```python
from build123d import *

# Parameters (mm, degrees)
BOSS_EXTRUDE1_DEPTH      = 60.1
BOSS_EXTRUDE1_DEPTH_BACK = 60.1
CUT_EXTRUDE3_DEPTH       = 86.526286164
CUT_EXTRUDE3_DEPTH_BACK  = 86.526286164
SKETCH2_R                = 3.34
CUT_EXTRUDE5_DEPTH       = 86.526286164
SKETCH8_R                = 5.08
CUT_EXTRUDE6_DEPTH       = 6.858


with BuildPart() as part:
    # Sketch5 → Boss-Extrude1 (new, two sides: drawn at the far end of the back side and taken through both)
    with BuildSketch(Plane(origin=(0, 0, 0), x_dir=(0, 0, -1), z_dir=(1, 0, 0)).offset(-BOSS_EXTRUDE1_DEPTH_BACK)):
        Polygon((60.1, 0), (-60.1, 0), (-54.75, 9.525), (54.75, 9.525), align=None)
    extrude(amount=BOSS_EXTRUDE1_DEPTH + BOSS_EXTRUDE1_DEPTH_BACK)

    # Sketch6 → Cut-Extrude3 (cut, two sides: drawn at the far end of the back side and taken through both)
    with BuildSketch(Plane.XY.offset(-CUT_EXTRUDE3_DEPTH_BACK)):
        Polygon((-54.75, 9.525), (-60.1, 0), (-60.1, 9.525), align=None)
        Polygon((60.1, 9.525), (54.75, 9.525), (60.1, 0), align=None)
    extrude(amount=CUT_EXTRUDE3_DEPTH + CUT_EXTRUDE3_DEPTH_BACK, mode=Mode.SUBTRACT)

    # Sketch2 → Cut-Extrude5 (cut, through all)
    with BuildSketch(Plane(origin=(0, 0, 0), x_dir=(1, 0, 0), z_dir=(0, 1, 0))):
        with Locations(Location((-25, 25, 0), (0, 0, 270))):
            Circle(SKETCH2_R)
        with Locations(Location((25, 25, 0), (0, 0, 270))):
            Circle(SKETCH2_R)
        with Locations(Location((25, -25, 0), (0, 0, 270))):
            Circle(SKETCH2_R)
        with Locations(Location((-25, -25, 0), (0, 0, 270))):
            Circle(SKETCH2_R)
        Polygon((-39.357563441, 0), (0, 39.357563441), (39.357563441, 0), (0, -39.357563441), align=None)
    extrude(amount=CUT_EXTRUDE5_DEPTH, mode=Mode.SUBTRACT)

    # Sketch8 → Cut-Extrude6 (cut)
    with BuildSketch(Plane.XZ):
        with Locations(Location((-25, 25, 0), (0, 0, 270))):
            Circle(SKETCH8_R)
        with Locations(Location((25, 25, 0), (0, 0, 270))):
            Circle(SKETCH8_R)
        with Locations(Location((25, -25, 0), (0, 0, 270))):
            Circle(SKETCH8_R)
        with Locations(Location((-25, -25, 0), (0, 0, 270))):
            Circle(SKETCH8_R)
    extrude(amount=-CUT_EXTRUDE6_DEPTH, mode=Mode.SUBTRACT)


solid = part.part
```
Here's how the part is built. I have some questions about the finished solid (model axes, mm). A direction names the side the tool comes from. Round coordinates to 2 decimals unless told otherwise and drop trailing zeros. Loops run counter-clockwise (first coordinate to the right, second up) from the corner with the lowest first, then second, coordinate; pieces in that order, holes last. Notation, with made-up numbers: (71, 74) -> (93, 74) arc R37 cw to (93, 112) -> close; hole circle Ø9 at (-17.5, 44). An arc over 180 degrees is marked (long way). Answer as CSV lines item,"result". Start each with the question number.
1. If we mould it in two halves opening along X, with no side actions, what happens to faces 4 (the face through (-37, 9.525, -11)), 5 (the face through (57.388, 4.829, -0.841)), 6 (the face through (-28.09, 3.38, -20.97))? For each: pulls with the +X half, pulls with the -X half, needs draft (parallel to the pull), parting line crosses it, or undercut.
2. Imagine slicing it at C-C on y = 2.5. Write out the boundary of the cut face in (x, z), plus the area to 3 significant figures.
3. For faces 1 (the face through (-0.84, 4.7, 57.46)), 2 (the face through (-28.3, 6.858, 26.2)), 3 (the face through (-19.954, 4.696, -19.403)), which set-ups out of +Z, -Z, +X, -X, +Y, -Y let a thin tool reach every point of the face, with its end or its side?
4. Imagine slicing it at B-B on x = -5. Write out the boundary of the cut face in (y, z) (3 decimals).
5. I need wall thicknesses on probe 1 along X at (y, z) = (5.25, -25); probe 2 along Z at (x, y) = (25, 9); probe 3 along X at (y, z) = (7.75, 25). Which ranges of each line are inside material? Lowest first, please. Write a range as from..to.
6. I'm going to push flat-ended pins straight in: P1, Ø2, axis at y = 2.5, z = 31, coming from the +X side; P2, Ø7.5, axis at x = 25, z = -25, coming from the -Y side; P3, Ø4, axis at y = 4.5, z = 13.5, coming from the -X side. Where does each tip first touch, or does it pass through?
7. Imagine slicing it at A-A on z = -16. Write out the boundary of the cut face in (x, y) (3 decimals).
8. Imagine slicing it at D-D on x = -25. Write out the boundary of the cut face in (y, z) (3 decimals), plus the area to 3 significant figures.
Solution:
1,face 4,"needs draft"
1,face 5,"pulls with the +X half"
1,face 6,"undercut"
2,outline,"(-58.7, -58.7) -> (58.7, -58.7) -> (58.7, 58.7) -> (-58.7, 58.7) -> close; hole (-39.36, 0) -> (0, -39.36) -> (39.36, 0) -> (0, 39.36) -> close; hole circle Ø10.16 at (-25, -25); hole circle Ø10.16 at (-25, 25); hole circle Ø10.16 at (25, -25); hole circle Ø10.16 at (25, 25)"
2,area,"10,400 mm²"
3,face 1,"+Z, +X, -X, +Y"
3,face 2,"-Y"
3,face 3,"+Y, -Y"
4,outline,"(0, -60.1) -> (9.525, -54.75) -> (9.525, -34.358) -> (0, -34.358) -> close; (0, 34.358) -> (9.525, 34.358) -> (9.525, 54.75) -> (0, 60.1) -> close"
5,probe 1,"-57.15..-30.08, -19.92..-14.36, 14.36..19.92, 30.08..57.15"
5,probe 2,"-55.04..-28.34, -21.66..-14.36, 14.36..21.66, 28.34..55.04"
5,probe 3,"-55.75..-28.34, -21.66..-14.36, 14.36..21.66, 28.34..55.75"
6,P1,"x = 59.26"
6,P2,"y = 6.86"
6,P3,"x = -58.7"
7,outline,"(-60.1, 0) -> (-23.358, 0) -> (-23.358, 9.525) -> (-54.75, 9.525) -> close; (23.358, 0) -> (60.1, 0) -> (54.75, 9.525) -> (23.358, 9.525) -> close"
8,outline,"(0, -60.1) -> (9.525, -54.75) -> (9.525, -28.34) -> (6.858, -28.34) -> (6.858, -30.08) -> (0, -30.08) -> close; (0, -19.92) -> (6.858, -19.92) -> (6.858, -21.66) -> (9.525, -21.66) -> (9.525, -14.358) -> (0, -14.358) -> close; (0, 14.358) -> (9.525, 14.358) -> (9.525, 21.66) -> (6.858, 21.66) -> (6.858, 19.92) -> (0, 19.92) -> close; (0, 30.08) -> (6.858, 30.08) -> (6.858, 28.34) -> (9.525, 28.34) -> (9.525, 54.75) -> (0, 60.1) -> close"
8,area,"645 mm²"
